from build123d import *

# Parameters (mm, degrees)
F1_DEPTH = 88.9
F2_R     = 4.7625
F3_DEPTH = 127.001
F5_DEPTH = 127.001


with BuildPart() as f1:
    # F0 (on Top) → F1 (new body)
    with BuildSketch(Plane.XY):
        Polygon((508, -63.5), (508, -44.45), (1828.8, -44.45), (1828.8, 44.45), (508, 44.45), (508, 63.5), (0, 63.5), (0, 44.45), (0, -44.45), (0, -63.5), align=None)
    extrude(amount=F1_DEPTH)

    # F2 (on face) → F3 (cut, through all)
    with BuildSketch(Plane.XZ.offset(63.5)):
        with Locations((44.45, 44.45)):
            Circle(F2_R)
        with Locations((304.8, 44.45)):
            Circle(F2_R)
        with Locations((406.4, 44.45)):
            Circle(F2_R)
    extrude(amount=-F3_DEPTH, mode=Mode.SUBTRACT)

    # F4 (on face) → F5 (cut, through all)
    with BuildSketch(Plane.XZ.offset(63.5)):
        with BuildLine():
            ThreePointArc((0, 0), (26.038207, 62.861793), (88.9, 88.9))
            Line((88.9, 88.9), (0, 88.9))
            Line((0, 88.9), (0, 0))
        make_face()
    extrude(amount=-F5_DEPTH, mode=Mode.SUBTRACT)


solid = f1.part
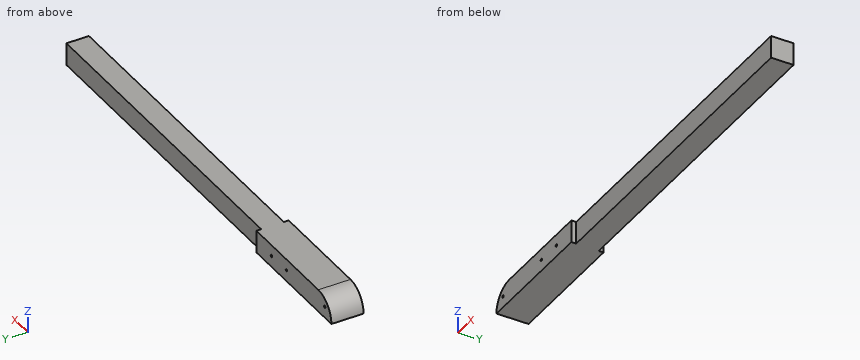
Geometry: final body of the model. Coordinates: model frame, mm. Coordinates: 2 decimals unless noted, no trailing zeros. Loops run counter-clockwise (first coordinate to the right, second up) from the corner with the lowest first, then second, coordinate; pieces in that order, holes last. Notation, with made-up numbers: M -36,79.5 L 1,79.5 A22 cw 1,105.5 Z; hole C 28.5,53.5 d4. An arc over 180 degrees is marked long. One line per item, written item: value. Start each with the question number.
1) Material intervals for L1, parallel to Z at x = 406, y = 8; L2, parallel to X at y = 23, z = 44; L3, parallel to X at y = -23, z = 45, sorted ascending. Write a range as from..to.
2) Pin query (flat end, axial travel): P1, Ø4, axis at x = 1331.5, z = 73, coming from the +Y side; P2, Ø9.5, axis at y = -50.5, z = 29.5, coming from the +X side; P3, Ø12, axis at x = 1073.5, z = 60, coming from the -Y side; P4, Ø7.5, axis at x = 304.8, z = 44.45, coming from the -Y side. Return the tip coordinate at first contact, or that it passes through.
3) Cut plane A-A (x = 1518). Return loops of the section in (y, z), then the cut area to 3 significant figures.
Evaluation:
1. L1: 0..39.7, 49.2..88.9
1. L2: 11.65..39.71, 49.19..300.06, 309.54..401.66, 411.14..1828.8
1. L3: 12.23..39.72, 49.18..300.07, 309.53..401.67, 411.13..1828.8
2. P1: y = 44.45
2. P2: x = 508
2. P3: y = -44.45
2. P4: through
3. outline: M -44.45,0 L 44.45,0 L 44.45,88.9 L -44.45,88.9 Z
3. area: 7,900 mm^2
